```python
from build123d import *

# Parameters (mm, degrees)
F0_R     = 5.982402
F1_DEPTH = 200
F2_W     = 45.446075
F2_H     = 2.038203
F3_DEPTH = 12.5
F4_R     = 61.03573
F5_DEPTH = 25
F6_W     = 51.913552
F6_H     = 32.489951
F7_DEPTH = 10


with BuildPart() as f1:
    # F0 (on Right) → F1 (new body)
    with BuildSketch(Plane.YZ):
        Circle(F0_R)
    extrude(amount=F1_DEPTH)

    # F2 (on Top) → F3 (cut, symmetric)
    with BuildSketch(Plane.XY):
        with Locations((22.723038, 5.091489)):
            Rectangle(F2_W, F2_H)
    extrude(amount=F3_DEPTH, both=True, mode=Mode.SUBTRACT)

    # F4 (on face) → F5 (cut)
    with BuildSketch(Plane(origin=(0, 4.072388, 0), x_dir=(-1, 0, 0), z_dir=(0, 1, 0))):
        with Locations((15.432127, 0)):
            Circle(F4_R)
    extrude(amount=F5_DEPTH, mode=Mode.SUBTRACT)

    # F6 (on face) → F7 (cut)
    with BuildSketch(Plane(origin=(0, 0, 0), x_dir=(0, -1, 0), z_dir=(-1, 0, 0))):
        with Locations((-6.045349, -2.592297)):
            Rectangle(F6_W, F6_H)
    extrude(amount=-F7_DEPTH, mode=Mode.SUBTRACT)


solid = f1.part
```
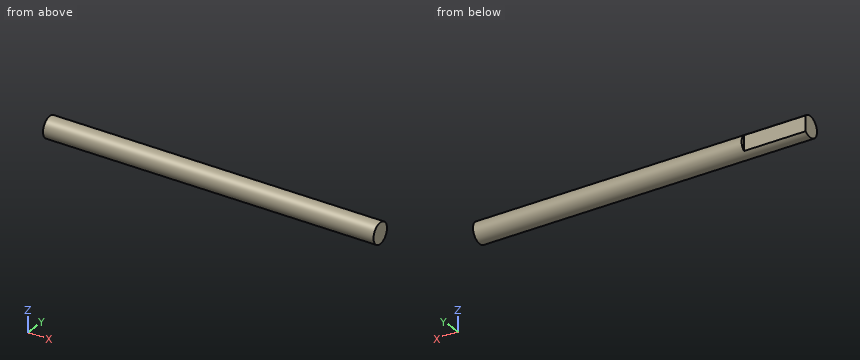
The listing builds one solid part. Answer for the finished solid, in the listing's coordinates (mm). Give positions to 0.01 mm unless a question says otherwise; leave off trailing zeros. Loops run counter-clockwise (first coordinate to the right, second up) from the corner with the lowest first, then second, coordinate; pieces in that order, holes last. Notation, with made-up numbers: (36, 18.25) - (61, 18.25) arc R25 ccw to (61, 51.25) - close; hole circle Ø11 at (75, 57). An arc over 180 degrees is marked (long way). Return JSON: item names as keys, results as strings. Group by question number.
1. Given pin 1 Ø3 at (x, y) = (93, -2) entering from -Z; pin 2 Ø1.5 at (x, y) = (141.5, -3) entering from -Z; pin 3 Ø5 at (x, y) = (73.5, -4) entering from -Z, each flat-ended and moving along its own axis, determine where each tip first touches the part or whether it passes through.
2. Find section B-B (x = 88). Write down the section's boundary in (y, z).
3. Straight lines are drawn through the part: line 1 (Y direction, x = 115, z = 0.25); line 2 (Z direction, x = 108, y = 0.5); line 3 (Z direction, x = 144.5, y = 4.25). For each, find the intervals that lie inside material, in ascending order. Write a range as [from, to].
4. Find section D-D (x = 29.5). Write down the section's boundary in (y, z).
5. Find section A-A (z = 0). Write down the section's boundary in (x, y), then the cut area to 3 significant figures.
6. Find section C-C (y = 2). Write down the section's boundary in (x, z), then the cut area to 3 significant figures.
Verdict:
{
 "1": {"pin 1": "stops at z = -5.96", "pin 2": "stops at z = -5.54", "pin 3": "stops at z = -5.79"},
 "2": {"outline": "circle Ø11.96 at (0, 0)"},
 "3": {"line 1": "y = [-5.98, 5.98]", "line 2": "z = [-5.96, 5.96]", "line 3": "z = [-4.21, 4.21]"},
 "4": {"outline": "(4.07, -4.38) - (4.07, 4.38) arc R5.98 ccw (long way) to start"},
 "5": {"outline": "(10, -5.98) - (200, -5.98) - (200, 5.98) - (45.6, 5.98) - (45.6, 4.07) - (10, 4.07) - close", "area": "2,210 mm^2"},
 "6": {"outline": "(10, -5.64) - (200, -5.64) - (200, 5.64) - (10, 5.64) - close", "area": "2,140 mm^2"}
}
